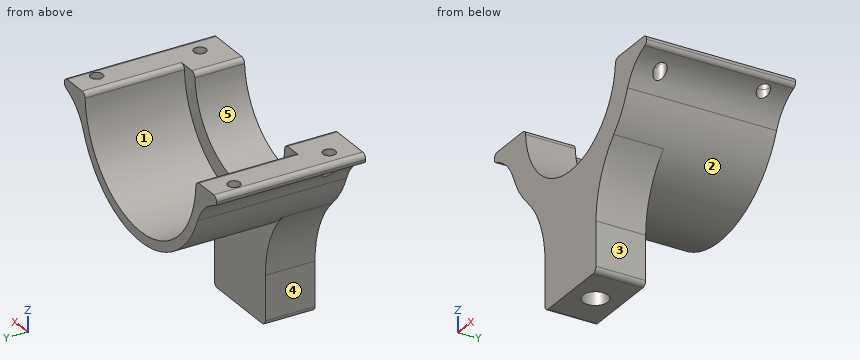
from build123d import *

# Parameters (mm, degrees)
ESQUISSE1_W                               = 17
ESQUISSE1_H                               = 10
BOSS_EXTRU_1_DEPTH                        = 20
TROUS_DE_CENTRAGE_5_0MM1_D                = 5
TROUS_DE_CENTRAGE_5_0MM1_DEPTH            = 10
TROUS_DE_CENTRAGE_5_0MM1_TIP              = 1.502151548
BOSS_EXTRU_2_DEPTH                        = 20
BOSS_EXTRU_3_START                        = 10
BOSS_EXTRU_3_DEPTH                        = 10
CONG_1_R                                  = 20
TROU_POUR_TARAUDAGE_POUR_TROU_TARAUD_M3_D = 2.5
CONG_2_R                                  = 1
CONG_3_START                              = -5
CONG_3_DEPTH                              = 30
CONG_3_START_2                            = 32
CONG_3_2_OUTLINE_R                        = 1.25
CONG_3_2_DEPTH                            = 4.654758106


with BuildPart() as part:
    # Esquisse1 → Boss.-Extru.1 (new body)
    with BuildSketch(Plane.XY):
        Rectangle(ESQUISSE1_W, ESQUISSE1_H)
    extrude(amount=BOSS_EXTRU_1_DEPTH)

    # Trous de centrage Ø5.0mm1
    with Locations(Plane(origin=(0, 0, 0), x_dir=(-1, 0, 0), z_dir=(0, 0, -1))):
        with Locations((0, 0)):
            Hole(TROUS_DE_CENTRAGE_5_0MM1_D / 2, depth=TROUS_DE_CENTRAGE_5_0MM1_DEPTH)
            with Locations((0, 0, -(TROUS_DE_CENTRAGE_5_0MM1_DEPTH + TROUS_DE_CENTRAGE_5_0MM1_TIP / 2))):  # 118° drill point
                Cone(0, TROUS_DE_CENTRAGE_5_0MM1_D / 2, TROUS_DE_CENTRAGE_5_0MM1_TIP, mode=Mode.SUBTRACT)

    # Esquisse4 → Boss.-Extru.2 (add)
    with BuildSketch(Plane(origin=(0, 5, 0), x_dir=(1, 0, 0), z_dir=(0, 1, 0))):
        with BuildLine():
            Line((18.5, -38.654758106), (25.402205763, -38.654758106))
            Line((25.402205763, -38.654758106), (25.402205763, -36.654758106))
            Line((25.402205763, -36.654758106), (20.402205763, -36.654758106))
            ThreePointArc((20.402205763, -36.654758106), (0, -18.154758106), (-20.402205763, -36.654758106))
            Line((-20.402205763, -36.654758106), (-25.402205763, -36.654758106))
            Line((-25.402205763, -36.654758106), (-25.402205763, -38.654758106))
            Line((-25.402205763, -38.654758106), (-18.5, -38.654758106))
            ThreePointArc((-18.5, -38.654758106), (0, -20.154758106), (18.5, -38.654758106))
        make_face()
    extrude(amount=BOSS_EXTRU_2_DEPTH)

    # Esquisse5 → Boss.-Extru.3 (add)
    with BuildSketch(Plane.XZ.offset(-5).offset(BOSS_EXTRU_3_START)):
        with BuildLine():
            Line((-18.5, 38.654758106), (-15, 38.654758106))
            ThreePointArc((-15, 38.654758106), (0, 23.654758106), (15, 38.654758106))
            Line((15, 38.654758106), (18.5, 38.654758106))
            Line((18.5, 38.654758106), (25.402205763, 38.654758106))
            Line((25.402205763, 38.654758106), (25.402205763, 36.654758106))
            Line((25.402205763, 36.654758106), (20.402205763, 36.654758106))
            ThreePointArc((20.402205763, 36.654758106), (16.678717468, 26.735429953), (8.5, 20))
            Line((8.5, 20), (-8.5, 20))
            ThreePointArc((-8.5, 20), (-16.678717468, 26.735429953), (-20.402205763, 36.654758106))
            Line((-20.402205763, 36.654758106), (-25.402205763, 36.654758106))
            Line((-25.402205763, 36.654758106), (-25.402205763, 38.654758106))
            Line((-25.402205763, 38.654758106), (-18.5, 38.654758106))
        make_face()
    extrude(amount=-BOSS_EXTRU_3_DEPTH)

    # Congé1
    cong_1_edges = [part.edges().sort_by_distance(p)[0] for p in [
        (-8.5, 0, 20),
        (8.5, 0, 20),
    ]]
    fillet(cong_1_edges, radius=CONG_1_R)

    # Trou pour taraudage pour trou taraudé M31 (through all)
    with Locations(Plane.XY.offset(38.654758106)):
        with Locations((-22.902205763, 20), (-21.551356318, 0), (21.551356318, 0), (22.902205763, 20)):
            Hole(TROU_POUR_TARAUDAGE_POUR_TROU_TARAUD_M3_D / 2)

    # Congé2
    cong_2_edges = [part.edges().sort_by_distance(p)[0] for p in [
        (-15, 0, 38.654758106),
        (-8.5, 0, 0),
        (8.5, 0, 0),
        (25.402205763, 10, 36.654758106),
        (-25.402205763, 10, 36.654758106),
        (25.402205763, 10, 38.654758106),
        (18.5, 15, 38.654758106),
        (-18.5, 15, 38.654758106),
        (15, 0, 38.654758106),
        (-25.402205763, 10, 38.654758106),
    ]]
    fillet(cong_2_edges, radius=CONG_2_R - 0.0001)  # a hair under: the kernel refuses the full size

    # Congé3: read off the stored shape, not the designer's step
    # Congé3 outline → Congé3 (add)
    with BuildSketch(Plane(origin=(0, 0, 0), x_dir=(1, 0, 0), z_dir=(0, 1, 0)).offset(CONG_3_START)):
        with BuildLine():
            ThreePointArc((-20.402205763, -36.654758106), (-19.921613651, -33.819542541), (-19.049016512, -31.079471318))
            ThreePointArc((-19.049016512, -31.079471318), (-21.313684521, -34.498543554), (-24.760297938, -36.721071866))
            ThreePointArc((-24.760297938, -36.721071866), (-24.584296071, -36.671476295), (-24.402205763, -36.654758106))
            Line((-24.402205763, -36.654758106), (-20.402205763, -36.654758106))
        make_face()
        with BuildLine():
            ThreePointArc((24.760297938, -36.721071866), (21.313684521, -34.498543554), (19.049016512, -31.079471318))
            ThreePointArc((19.049016512, -31.079471318), (19.921613651, -33.819542541), (20.402205763, -36.654758106))
            Line((20.402205763, -36.654758106), (24.402205763, -36.654758106))
            ThreePointArc((24.402205763, -36.654758106), (24.584296071, -36.671476295), (24.760297938, -36.721071866))
        make_face()
    extrude(amount=CONG_3_DEPTH)

    # Cong_3 2 outline → Cong_3 2 (cut)
    with BuildSketch(Plane.XY.offset(CONG_3_START_2)):
        with Locations((22.902205763, 20)):
            Circle(CONG_3_2_OUTLINE_R)
        with Locations((21.551356318, 0)):
            Circle(CONG_3_2_OUTLINE_R)
        with Locations((-21.551356318, 0)):
            Circle(CONG_3_2_OUTLINE_R)
        with Locations((-22.902205763, 20)):
            Circle(CONG_3_2_OUTLINE_R)
    extrude(amount=CONG_3_2_DEPTH, mode=Mode.SUBTRACT)


solid = part.part
Source: CAD feature listing. Evaluate the final solid. Frame: model axes, mm. Face numbers are marked on the shaded views. A direction names the side the tool comes from. Coordinates: 2 decimals unless noted, no trailing zeros. Order: outer loops, then holes, each group sorted by start corner. A loop starts at its lowest first (then second) coordinate and runs counter-clockwise, first axis right, second up. Notation, with made-up numbers: M 48,79.5 L 103,79.5 A25 ccw 103,96.5 Z; hole C 37,53 d3. An arc over 180 degrees is marked long. Write each question's results on one line, items separated by ' | '. Start each with the question number.
Item 1: Cut plane A-A (y = 20). Count the separate pieces of the cut face and the enclosed holes in it, and give its area (3 significant figures).
Item 2: Line query: probe 1 along X at (y, z) = (0, 8); probe 2 along Y at (x, z) = (-16, 30); probe 3 along X at (y, z) = (20, 35.8). Output: solid intervals per line, ascending.
Item 3: First-contact query: pin 1 Ø4 at (x, y) = (21.55, 0) entering from -Z; pin 2 Ø5 at (x, y) = (5, 10) entering from +Z; pin 3 Ø1.5 at (x, y) = (-21.55, 0) entering from +Z; pin 4 Ø2 at (x, y) = (-5, 12) entering from -Z. Flat tips, straight axial feed; report the tip coordinate or a pass-through.
Item 4: Set-up query: the marked faces 1, 2, 3, 4 and 5. Return all of +Z, -Z, +X, -X, +Y, -Y with unobstructed straight access to the full face (end or side cutting, diameter ignored); none if empty.
Item 5: Cut plane C-C (x = -13). Return loops of the section in (y, z), and give its area (3 significant figures).
Item 6: Cut plane B-B (z = 5.5). Return loops of the section in (x, y).
Item 7: Cut plane D-D (z = 29). Return loops of the section in (x, y).
Checked values:
1) separate pieces: 3 | enclosed holes: 0 | area: 140 mm2
2) probe 1: x = -8.5 to -2.5, 2.5 to 8.5 | probe 2: y = -5 to 5 | probe 3: x = -21.65 to -18.28, 18.28 to 21.65
3) pin 1: stops at z = 32.15 | pin 2: stops at z = 21.74 | pin 3: passes through | pin 4: stops at z = 18.55
4) face 1: +Z, +Y | face 2: -Z, +Y | face 3: -Z, +X, +Y, -Y | face 4: -Z, -X, +Y, -Y | face 5: +Z, +Y, -Y
5) outline: M -5,22.52 L 5,22.52 L 5,22.8 L 25,22.8 L 25,25.49 L 5,25.49 L 5,31.17 L -5,31.17 Z | area: 140 mm2
6) outline: M -8.5,-5 L 8.5,-5 L 8.5,5 L -8.5,5 Z; hole C 0,0 d5
7) outline: M -18.08,-5 L -11.48,-5 L -11.48,5 L -15.78,5 L -15.78,25 L -18.08,25 Z; M 11.48,-5 L 18.08,-5 L 18.08,25 L 15.78,25 L 15.78,5 L 11.48,5 Z
